The model under review builds one solid part; all positions refer to its coordinate system, in mm. A direction names the side the tool comes from. Round coordinates to 2 decimals unless told otherwise and drop trailing zeros. Order: outer loops, then holes, each group sorted by start corner. A loop starts at its lowest first (then second) coordinate and runs counter-clockwise, first axis right, second up. Notation, with made-up numbers: M 20,-18.75 L 64,-18.75 A22 ccw 64,6.25 Z; hole C 45.25,30.25 d7. An arc over 180 degrees is marked long. Use a Markdown table: item, result. Add a question column.
1. Insertion check: P1, Ø4, axis at x = 16, z = -20.5, coming from the -Y side; P2, Ø8, axis at x = 59, z = -23.5, coming from the +Y side. Each pin has a flat end and moves straight along its axis. Give the tip position at first contact, or say it passes through.
2. Consider section A-A on x = 24.5. State the section outline as (y, z) points, then the cut area to 3 significant figures.
3. The part is to be moulded in two halves that separate along Z. For faces 3 (the flat face through (93.1, -11.55, -37.5)), 4 (the flat face through (3.66, -11.12, -2.85)), 5 (the flat face through (92.86, -11.12, -37.73)), say which applies: +Z half, -Z half, draft (parallel to the pull), parting line (faces both ways), or undercut.
4. To check wall thickness, follow probe 1 along X at (y, z) = (0.5, -25); probe 2 along Y at (x, z) = (10.5, -5); probe 3 along Y at (x, z) = (77, -21). State the ranges of each line that lie inside material, in increasing order.
5. Consider section B-B on z = -21.5. State the section outline as (x, y) points, then the cut area to 3 significant figures.
6. For faces 1 (the flat face through (3.66, -11.12, -37.15)), 2 (the flat face through (32.14, -11.12, -2.27)), list the 3-axis set-ups (+Z, -Z, +X, -X, +Y, -Y) from which the entire face can be reached by the end or side of a thin tool; tool diameter is ignored.
from build123d import *

# Parameters (mm, degrees)
SKETCH1_W           = 97
SKETCH1_H           = 40
SKETCH1_W_2         = 76.4
SKETCH1_H_2         = 26.8
BOSS_EXTRUDE2_DEPTH = 1
FILLET1_R           = 0.2
SKETCH2_W           = 97
SKETCH2_H           = 40
BOSS_EXTRUDE3_DEPTH = 9.3
LPATTERN1_COUNT     = 2
LPATTERN1_PITCH     = 28


# Read off the part's stored shape, not the designer's step: Mirror1, Mirror2
with BuildPart() as part:
    # Sketch1 → Boss-Extrude2 (new body)
    with BuildSketch(Plane(origin=(0, 0, 0), x_dir=(1, 0, 0), z_dir=(0, 1, 0))):
        with Locations((48.5, 20)):
            Rectangle(SKETCH1_W, SKETCH1_H)
        with Locations((48.5, 20)):
            Rectangle(SKETCH1_W_2, SKETCH1_H_2, mode=Mode.SUBTRACT)
        with BuildLine():
            Line((4.3, 37.75), (92.7, 37.75))
            ThreePointArc((92.7, 37.75), (93.075, 37.375), (92.7, 37))
            Line((92.7, 37), (4.3, 37))
            ThreePointArc((4.3, 37), (3.925, 37.375), (4.3, 37.75))
        make_face(mode=Mode.SUBTRACT)
        with BuildLine():
            Line((4.3, 2.25), (92.7, 2.25))
            ThreePointArc((92.7, 2.25), (93.075, 2.625), (92.7, 3))
            Line((92.7, 3), (4.3, 3))
            ThreePointArc((4.3, 3), (3.925, 2.625), (4.3, 2.25))
        make_face(mode=Mode.SUBTRACT)
    extrude(amount=BOSS_EXTRUDE2_DEPTH)

    # Fillet1
    fillet1_edges = [part.edges().sort_by_distance(p)[0] for p in [
        (3.925, 1, -37.375),
        (48.5, 1, -37),
        (93.075, 1, -37.375),
        (48.5, 1, -37.75),
        (3.925, 1, -2.625),
        (48.5, 1, -2.25),
        (93.075, 1, -2.625),
        (48.5, 1, -3),
    ]]
    fillet(fillet1_edges, radius=FILLET1_R)

    # Sketch2 → Boss-Extrude3 (add)
    with BuildSketch(Plane.XZ):
        with Locations((48.5, -20)):
            Rectangle(SKETCH2_W, SKETCH2_H)
    extrude(amount=BOSS_EXTRUDE3_DEPTH)

    # Sketch3 → Loft1 section 0
    with BuildSketch(Plane.XZ.offset(9.3)):
        with BuildLine():
            Line((2, 0), (3.5, 0))
            Line((3.5, 0), (3.5, -0.7))
            Line((3.5, -0.7), (2, -0.7))
            Line((2, -0.7), (2, 0))
        make_face()
    # Sketch5 → Loft1 section 1
    with BuildSketch(Plane(origin=(0, -10.7, 0), x_dir=(-1, 0, 0), z_dir=(0, -1, 0))):
        with BuildLine():
            Line((-2.4, 0.530034721), (-3.460660172, 1.590694893))
            Line((-3.460660172, 1.590694893), (-2.930330086, 2.121024979))
            Line((-2.930330086, 2.121024979), (-1.869669914, 1.060364807))
            Line((-1.869669914, 1.060364807), (-2.4, 0.530034721))
        make_face()
    loft1 = loft()

    # Sketch4 → Loft2 section 0
    with BuildSketch(Plane(origin=(0, -11.55, 0), x_dir=(-1, 0, 0), z_dir=(0, -1, 0))):
        with BuildLine():
            Line((-2.4, 0.530034721), (-5.935533906, 4.065568627))
            Line((-5.935533906, 4.065568627), (-5.40520382, 4.595898713))
            Line((-5.40520382, 4.595898713), (-1.869669914, 1.060364807))
            Line((-1.869669914, 1.060364807), (-2.4, 0.530034721))
        make_face()
    # Sketch6 → Loft2 section 1
    with BuildSketch(Plane(origin=(0, -10.7, 0), x_dir=(-1, 0, 0), z_dir=(0, -1, 0))):
        with BuildLine():
            Line((-5.935533906, 4.065568627), (-5.40520382, 4.595898713))
            Line((-5.40520382, 4.595898713), (-1.869669914, 1.060364807))
            Line((-1.869669914, 1.060364807), (-2.4, 0.530034721))
            Line((-2.4, 0.530034721), (-5.935533906, 4.065568627))
        make_face()
    loft2 = loft()

    # LPattern1: Loft1, Loft2 ×2
    with Locations(*[(i * LPATTERN1_PITCH, 0, 0) for i in range(1, LPATTERN1_COUNT)]):
        add(loft1)
        add(loft2)

    # Mirror1: part across plane


with BuildPart() as part_1:
    add(part.part)
    add(part.part.mirror(Plane(origin=(48.5, 0, 0), x_dir=(0, 0, 1), z_dir=(1, 0, 0))))

    # Mirror2: part across plane


with BuildPart() as part_2:
    add(part_1.part)
    add(part_1.part.mirror(Plane.XY.offset(-20)))


solid = part_2.part
Answer block:
| question | item | result |
|---|---|---|
| 1 | P1 | y = -9.3 |
| 1 | P2 | y = 0 |
| 2 | outline | M -9.3,-40 L 1,-40 L 1,-37.95 A0.2 ccw 0.8,-37.75 L 0,-37.75 L 0,-37 L 0.8,-37 A0.2 ccw 1,-36.8 L 1,-33.4 L 0,-33.4 L 0,-6.6 L 1,-6.6 L 1,-3.2 A0.2 ccw 0.8,-3 L 0,-3 L 0,-2.25 L 0.8,-2.25 A0.2 ccw 1,-2.05 L 1,0 L -9.3,0 Z |
| 2 | area | 384 mm^2 |
| 3 | face 3 | draft |
| 3 | face 4 | undercut |
| 3 | face 5 | -Z half |
| 4 | probe 1 | 0 to 10.3, 86.7 to 97 |
| 4 | probe 2 | -9.3 to 1 |
| 4 | probe 3 | -9.3 to 0 |
| 5 | outline | M 0,-9.3 L 97,-9.3 L 97,1 L 86.7,1 L 86.7,0 L 10.3,0 L 10.3,1 L 0,1 Z |
| 5 | area | 923 mm^2 |
| 6 | face 1 | -X, -Y |
| 6 | face 2 | +Z, -Y |
